```python
from build123d import *

# Parameters (mm, degrees)
CYLINDER_R        = 76.2
CYLINDER_DEPTH    = 10.668
BOX010_W          = 609.6
BOX010_H          = 10.668
BOX010_DEPTH      = 537.464
BOX010_ROLL_ANGLE = -90.0000000001


with BuildPart() as cablecutout:
    # Cylinder → Cylinder (new body)
    with BuildSketch(Plane(origin=(304.8, 304.8, 598.932), x_dir=(1, 0, 0), z_dir=(0, 0, 1))):
        Circle(CYLINDER_R)
    extrude(amount=CYLINDER_DEPTH)


with BuildPart() as centersupport:
    # Box010 → Box010 (new body)
    with BuildSketch(Plane.XY):
        with Locations((304.8, 5.334)):
            Rectangle(BOX010_W, BOX010_H)
    extrude(amount=BOX010_DEPTH)


with BuildPart() as centersupport_1:
    # Box010 roll: moved
    add(centersupport.part.rotate(Axis((0, 0, 0), (1, 0, 0)), BOX010_ROLL_ANGLE))


with BuildPart() as centersupport_2:
    # Box010 placement: moved
    add(centersupport_1.part.moved(Location((10.668, 36.068, 609.6))))

    # Cut: cut CableCutout
    add(cablecutout.part, mode=Mode.SUBTRACT)


solid = centersupport_2.part
```
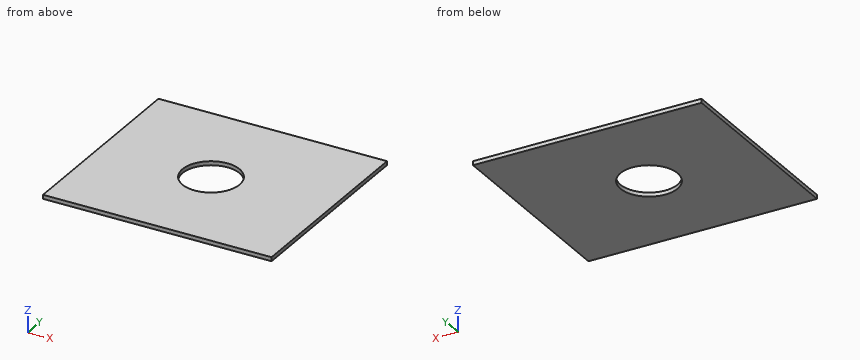
Geometry check sheet. Reference: the model listing, model coordinates, mm. Give positions to 0.01 mm unless a question says otherwise; leave off trailing zeros. Order: outer loops, then holes, each group sorted by start corner. A loop starts at its lowest first (then second) coordinate and runs counter-clockwise, first axis right, second up. Notation, with made-up numbers: (23.25, 27) - (53.25, 27) arc R22 ccw to (53.25, 59) - close; hole circle Ø10 at (3, -3). An arc over 180 degrees is marked (long way). Answer in a Markdown table with one row per item. Add a question column.
Q1. Cross-section at A-A, the plane x = 304.8. Enter the section's corners in (y, z), then the cut area to 3 significant figures.
Q2. Cross-section at C-C, the plane z = 607. Enter the section's corners in (x, y), then the cut area to 3 significant figures.
Q3. Cross-section at B-B, the plane y = 304.8. Enter the section's corners in (x, z).
Q4. Material ranges on probe 1 along Y at (x, z) = (304.8, 602.5); probe 2 along Y at (x, z) = (371.5, 604); probe 3 along X at (y, z) = (263.5, 605.5), recorded low to high. Write a range as from..to.
Check values:
| question | item | result |
|---|---|---|
| 1 | outline | (36.07, 598.93) - (228.6, 598.93) - (228.6, 609.6) - (36.07, 609.6) - close; (381, 598.93) - (573.53, 598.93) - (573.53, 609.6) - (381, 609.6) - close |
| 1 | area | 4,110 mm^2 |
| 2 | outline | (10.67, 36.07) - (620.27, 36.07) - (620.27, 573.53) - (10.67, 573.53) - close; hole circle Ø152.4 at (304.8, 304.8) |
| 2 | area | 309,000 mm^2 |
| 3 | outline | (10.67, 598.93) - (228.6, 598.93) - (228.6, 609.6) - (10.67, 609.6) - close; (381, 598.93) - (620.27, 598.93) - (620.27, 609.6) - (381, 609.6) - close |
| 4 | probe 1 | y = 36.07..228.6, 381..573.53 |
| 4 | probe 2 | y = 36.07..267.96, 341.64..573.53 |
| 4 | probe 3 | x = 10.67..240.76, 368.84..620.27 |
